The listing builds one solid part. Answer for the finished solid, in the listing's coordinates (mm). A direction names the side the tool comes from. Round coordinates to 2 decimals unless told otherwise and drop trailing zeros. Loops run counter-clockwise (first coordinate to the right, second up) from the corner with the lowest first, then second, coordinate; pieces in that order, holes last. Notation, with made-up numbers: M 8.5,69 L 31.5,69 A14 ccw 31.5,94 Z; hole C 39.5,44 d4. An arc over 180 degrees is marked long. Answer as a JSON object with one key per item and string values.
```python
from build123d import *

# Parameters (mm, degrees)
SKETCH1_R           = 12.5
SKETCH1_R_2         = 4.25
BOSS_EXTRUDE1_DEPTH = 5
BOSS_EXTRUDE2_START = -1
SKETCH2_R           = 4.25
BOSS_EXTRUDE2_DEPTH = 1
SKETCH3_R           = 1.25
CUT_EXTRUDE1_DEPTH  = 3
CHAMFER1_SIZE       = 1
CHAMFER1_SIZE2      = 1.428148007
FILLET1_R           = 2


with BuildPart() as part:
    # Sketch1 → Boss-Extrude1 (new body)
    with BuildSketch(Plane(origin=(0, 0, 0), x_dir=(1, 0, 0), z_dir=(0, 1, 0))):
        with Locations(Location((0, 0, 0), (0, 0, 270))):
            Circle(SKETCH1_R)
        with Locations(Location((0, 0, 0), (0, 0, 270))):
            Circle(SKETCH1_R_2, mode=Mode.SUBTRACT)
    extrude(amount=BOSS_EXTRUDE1_DEPTH)

    # Sketch2 → Boss-Extrude2 (add)
    with BuildSketch(Plane(origin=(0, 5, 0), x_dir=(1, 0, 0), z_dir=(0, 1, 0)).offset(BOSS_EXTRUDE2_START)):
        with Locations(Location((0, 0, 0), (0, 0, 270))):
            Circle(SKETCH2_R)
    extrude(amount=BOSS_EXTRUDE2_DEPTH)

    # Sketch3 → Cut-Extrude1 (cut)
    with BuildSketch(Plane(origin=(0, 0, 0), x_dir=(-1, 0, 0), z_dir=(0, -1, 0))):
        with Locations(Location((0, -9, 0), (0, 0, 90))):
            Circle(SKETCH3_R)
        with Locations(Location((-9, 0, 0), (0, 0, 90))):
            Circle(SKETCH3_R)
        with Locations(Location((0, 9, 0), (0, 0, 90))):
            Circle(SKETCH3_R)
        with Locations(Location((9, 0, 0), (0, 0, 90))):
            Circle(SKETCH3_R)
    extrude(amount=-CUT_EXTRUDE1_DEPTH, mode=Mode.SUBTRACT)

    # Chamfer1
    chamfer1_edges = [part.edges().sort_by_distance(p)[0] for p in [
        (0, 5, -12.5),
    ]]
    chamfer1_side = [part.faces().sort_by_distance(p)[0] for p in [
        (0, 2.5, -12.5),
    ]]
    chamfer(chamfer1_edges, length=CHAMFER1_SIZE, length2=CHAMFER1_SIZE2, reference=chamfer1_side[0])

    # Fillet1
    fillet1_edges = [part.edges().sort_by_distance(p)[0] for p in [
        (0, 5, -11.071851993),
        (0, 4, -12.5),
    ]]
    fillet(fillet1_edges, radius=FILLET1_R)


solid = part.part
```
Item 1: The part is cut by section A-A (y = 0.6). Give the vertices of the cut face in (x, z).
Values follow:
{"outline": "C 0,0 d25; hole C -9,0 d2.5; hole C 0,0 d8.5; hole C 0,-9 d2.5; hole C 0,9 d2.5; hole C 9,0 d2.5"}
Item 2: Flat-ended cylindrical pins translate along their axes: P1, Ø0.8, axis at x = 0, z = -8.5, coming from the -Y side; P2, Ø1, axis at y = 4.5, z = 9.5, coming from the -X side; P3, Ø2.5, axis at x = -1, z = 0, coming from the -Y side. Find the tip coordinate at first contact, or state that the pin passes through.
Values follow:
{"P1": "y = 3", "P2": "x = -7.94", "P3": "y = 4"}
Item 3: Which of the six approach directions +Z, -Z, +X, -X, +Y, -Y give full straight-line access (tool end or side, diameter ignored) to faces 1 (the face through (-5, 0, 0)), 2 (the face through (4.214, 1.972, -0.553))?
Values follow:
{"face 1": "+Z, -Z, +X, -X, -Y", "face 2": "-Y"}
Item 4: Straight lines are drawn through the part: line 1 (X direction, y = 0.65, z = 0); line 2 (Z direction, x = 0.75, y = 2.6); line 3 (Z direction, x = 2, y = 3.9). For each, find the intervals that lie inside material, in ascending order.
Values follow:
{"line 1": "-12.5 to -10.25, -7.75 to -4.25, 4.25 to 7.75, 10.25 to 12.5", "line 2": "-12.48 to -10, -8 to -4.18, 4.18 to 8, 10 to 12.48", "line 3": "-12.1 to -3.75, 3.75 to 12.1"}
Item 5: Determine the mould class of faces 3 (the face through (0, 5, 0)), 4 (the face through (-4.788, 1.459, 11.547)), 5 (the face through (-7.76, 1.48, 0.16)) for opening direction X: released by +X, released by -X, zero draft, split by the parting line, or undercut.
Values follow:
{"face 3": "zero draft", "face 4": "split by the parting line", "face 5": "undercut"}
